Design review of the part built by this model. Coordinates are the model's own, in mm. A direction names the side the tool comes from. Round coordinates to 2 decimals unless told otherwise and drop trailing zeros. Order: outer loops, then holes, each group sorted by start corner. A loop starts at its lowest first (then second) coordinate and runs counter-clockwise, first axis right, second up.
Autodesk Inventor part; units mm, degrees
ref_plane "YZ Plane" through (0, 0, 0) normal (1, 0, 0) x (0, 1, 0)
ref_plane "XZ Plane" through (0, 0, 0) normal (0, 1, 0) x (-1, 0, 0)
ref_plane "XY Plane" through (0, 0, 0) normal (0, 0, 1) x (1, 0, 0)
sketch "스케치1" plane through (0, 0, 0) normal (0, 1, 0) x (-1, 0, 0)
  line L0 (41, 0) -> (41, -21)
  line L1 (41, -21) -> (0, -21)
  line L2 (0, -21) -> (0, 0)
  line L3 (-4, -25) -> (45, -25)
  line L4 (45, -25) -> (45, 4)
  line L5 (-4, 4) -> (-4, -25)
  line L6 (41, -21) -> (0, -21)
  line L7 (30, 0) -> (30, 4)
  line L8 (11, 0) -> (11, 4)
  line L9 (0, 0) -> (11, 0)
  line L10 (30, 0) -> (41, 0)
  line L11 (45, 4) -> (30, 4)
  line L12 (11, 4) -> (-4, 4)
  line L13 (41, 0) -> (30, 0)
  line L14 (11, 0) -> (0, 0)
  dimension "d0" = 41
  dimension "d1" = 21
  dimension "d2" = 4
  dimension "d3" = 15
  dimension "d4" = 15
extrude "돌출1" add sketch "스케치1" along normal blind 40
ref_plane "작업 평면1" through (0, 20, 0) normal (0, 1, 0) x (1, 0, 0)
sketch "스케치3" plane through (0, 20, 0) normal (0, 1, 0) x (1, 0, 0)
  line L0 (-10.5, 25) -> (-10.5, 35)
  line L1 (-10.5, 35) -> (-30.5, 35)
  line L2 (-30.5, 35) -> (-30.5, 25)
  line L3 (4, 25) -> (-45, 25)
  line L4 (-20.5, 25) -> (-10.5, 35) construction
  line L5 (-20.5, 25) -> (-30.5, 35) construction
  point P0 (0, 0)
  dimension "d12" = 20
extrude "돌출2" add sketch "스케치3" along normal blind 15 and the other way blind 15
sketch "스케치4" plane through (-10.5, 35, -35) normal (0, 0, -1) x (-1, 0, 0)
  line L0 (20, 0) -> (20, -30)
  line L1 (0, 0) -> (20, 0)
  line L2 (0, -30) -> (0, 0)
  line L3 (20, -30) -> (0, -30)
  line L4 (0, 0) -> (20, 0)
  line L5 (16.6, -39.6) -> (3.4, -39.6)
  line L6 (3.4, -39.6) -> (3.4, 0)
  line L7 (3.4, 0) -> (16.6, 0)
  line L8 (16.6, 0) -> (16.6, -39.6)
  line L9 (16.6, -39.6) -> (3.4, 0) construction
  line L10 (3.4, -39.6) -> (16.6, 0) construction
  point P0 (-10.5, -35)
  point P1 (10, -19.8)
  point P2 (16.6, -30)
  point P3 (16.6, 0)
  point P4 (3.4, -30)
  point P5 (10, 0)
  dimension "d18" = 13.2
extrude "돌출3" cut sketch "스케치4" against normal blind 10 contours L8 L3 L6 L1
fillet "모깎기1" radius 2 8 edges at (-30.5, 20, -35) (-10.5, 20, -35) (-10.5, 20, -25) (-30.5, 20, -25) (-45, 20, -25) (4, 20, -25) (4, 20, 4) (-45, 20, 4)
properties part number "지그1"
1) Take a section at B-B on z = -31. Give the boundary of the cut face in (x, y).
Results:
outline: (-30.5, 5) - (-27.1, 5) - (-27.1, 35) - (-30.5, 35) - close; (-13.9, 5) - (-10.5, 5) - (-10.5, 35) - (-13.9, 35) - close
2) Clearance check with flat-ended pins moving along their axes: P1, Ø6, axis at x = -36, y = 17.5, coming from the -Z side; P2, Ø2.5, axis at x = -29, z = -32.5, coming from the +Y side; P3, Ø2.5, axis at x = -10.5, z = -29.5, coming from the -Y side. State where each tip first meets the part, or that it passes through.
Results:
P1: stops at z = -25
P2: stops at y = 35
P3: stops at y = 5
3) For faces 5 (the face through (-12, 35, -30)), 6 (the face through (-35, 20, 0)), 7 (the face through (-13.9, 20, -30)), 8 (the face through (-12, 5, -30)), 9 (the face through (-11, 20, 2)), list the 3-axis set-ups (+Z, -Z, +X, -X, +Y, -Y) from which the entire face can be reached by the end or side of a thin tool; tool diameter is ignored.
Results:
face 5: -Z, +X, -X, +Y
face 6: +Y, -Y
face 7: -Z, +Y, -Y
face 8: -Z, +X, -X, -Y
face 9: +Z, +Y, -Y
4) The part is to be moulded in two halves that separate along X. For faces 1 (the face through (-21, 20, -21)), 2 (the face through (-5, 20, 4)), 3 (the face through (-27.1, 20, -30)), 4 (the face through (-11.07, 20.21, -34.4)), say which applies: released by +X, released by -X, zero draft, split by the parting line, or undercut.
Results:
face 1: undercut
face 2: zero draft
face 3: undercut
face 4: released by +X
5) Take a section at D-D on x = -16. Give the boundary of the cut face in (y, z), plus the area to 3 significant figures.
Results:
outline: (0, -25) - (40, -25) - (40, -21) - (0, -21) - close
area: 160 mm2
6) To check wall thickness, follow line 1 along Z through (x, y) = (-34, 29.5); line 2 along X through (y, z) = (23, -31.5); line 3 along X through (y, z) = (36.5, 1). State the ranges of each line that lie inside material, in increasing order.
Results:
line 1: z = -25 to -21, 0 to 4
line 2: x = -30.5 to -27.1, -13.9 to -10.5
line 3: x = -45 to -30, -11 to 4
7) Take a section at C-C on y = 24.5. Give the boundary of the cut face in (x, z).
Results:
outline: (-45, -23) arc R2 ccw to (-43, -25) - (-32.5, -25) arc R2 cw to (-30.5, -27) - (-30.5, -33) arc R2 ccw to (-28.5, -35) - (-27.1, -35) - (-27.1, -25) - (-13.9, -25) - (-13.9, -35) - (-12.5, -35) arc R2 ccw to (-10.5, -33) - (-10.5, -27) arc R2 cw to (-8.5, -25) - (2, -25) arc R2 ccw to (4, -23) - (4, 2) arc R2 ccw to (2, 4) - (-11, 4) - (-11, 0) - (0, 0) - (0, -21) - (-41, -21) - (-41, 0) - (-30, 0) - (-30, 4) - (-43, 4) arc R2 ccw to (-45, 2) - close
8) Take a section at A-A on x = -35. Give the boundary of the cut face in (y, z).
Results:
outline: (0, -25) - (40, -25) - (40, -21) - (0, -21) - close; (0, 0) - (40, 0) - (40, 4) - (0, 4) - close
